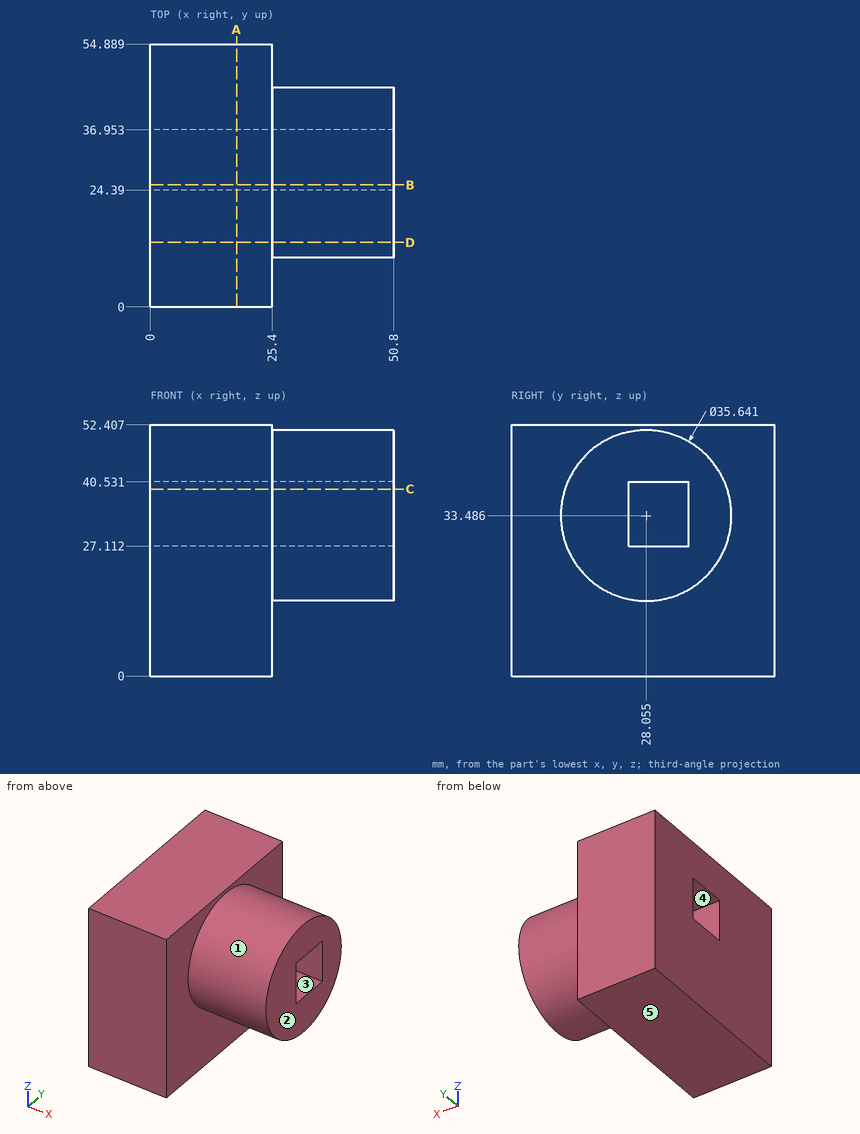
The drawing under review shows one solid part. Ordinate dimensions are in mm from its lowest x, y, z. A direction names the side the tool comes from. Round coordinates to 2 decimals unless told otherwise and drop trailing zeros. Order: outer loops, then holes, each group sorted by start corner. A loop starts at its lowest first (then second) coordinate and runs counter-clockwise, first axis right, second up. Notation, with made-up numbers: (-30, 6) -> (-2, 6) arc R21 ccw to (-2, 16) -> close; hole circle Ø4 at (-11, 1). An arc over 180 degrees is marked (long way). Return JSON: item names as keys, results as strings.
1. For the marked faces 4 and 5, list the 3-axis set-ups (+Z, -Z, +X, -X, +Y, -Y) from which the entire face can be reached by the end or side of a thin tool; tool diameter is ignored.
Answer block:
{"face 4": "+X, -X", "face 5": "-Z, +X, -X, +Y, -Y"}
2. The part is to be moulded in two halves that separate along Z. For the marked faces 1, 2 and 3, say which applies: +Z half, -Z half, draft (parallel to the pull), parting line (faces both ways), or undercut.
Answer block:
{"face 1": "parting line", "face 2": "draft", "face 3": "undercut"}
3. Take a section at B-B (y = 25.5). Write out the cut boundary in (x, z), then the cut area to 3 significant figures.
Answer block:
{"outline": "(0, 0) -> (25.4, 0) -> (25.4, 15.85) -> (50.8, 15.85) -> (50.8, 27.11) -> (0, 27.11) -> close; (0, 40.53) -> (50.8, 40.53) -> (50.8, 51.12) -> (25.4, 51.12) -> (25.4, 52.41) -> (0, 52.41) -> close", "area": "1,550 mm²"}
4. Take a section at D-D (y = 13.5). Write out the cut boundary in (x, z).
Answer block:
{"outline": "(0, 0) -> (25.4, 0) -> (25.4, 23.2) -> (50.8, 23.2) -> (50.8, 43.77) -> (25.4, 43.77) -> (25.4, 52.41) -> (0, 52.41) -> close"}
5. Take a section at C-C (z = 39). Write out the cut boundary in (x, y).
Answer block:
{"outline": "(0, 0) -> (25.4, 0) -> (25.4, 11.11) -> (50.8, 11.11) -> (50.8, 24.39) -> (0, 24.39) -> close; (0, 36.95) -> (50.8, 36.95) -> (50.8, 45) -> (25.4, 45) -> (25.4, 54.89) -> (0, 54.89) -> close"}
6. For L1, parallel to Z at x = 16, y = 27; L2, parallel to Y at x = 18, z = 28; L3, parallel to X at y = 49, z = 15.5, list the stretches that pass through material, from the lowest coordinate up. Write a range as [from, to].
Answer block:
{"L1": "z = [0, 27.11], [40.53, 52.41]", "L2": "y = [0, 24.39], [36.95, 54.89]", "L3": "x = [0, 25.4]"}
7. Insertion check: P1, Ø10, axis at x = 28.5, y = 32, coming from the +Z side; P2, Ø4, axis at x = 30, z = 31.5, coming from the -Y side (1 decimal); P3, Ø2, axis at y = 5.5, z = 11, coming from the +X side; P4, Ø1.5, axis at x = 45.5, y = 13.5, coming from the -Z side (1 decimal). Each pin has a flat end and moves straight along its axis. Give the tip position at first contact, or say it passes through.
Answer block:
{"P1": "stops at z = 52.41", "P2": "stops at y = 10.2", "P3": "stops at x = 25.4", "P4": "stops at z = 22.2"}
8. Take a section at A-A (x = 18). Write out the cut boundary in (y, z), then the cut area to 3 significant figures.
Answer block:
{"outline": "(0, 0) -> (54.89, 0) -> (54.89, 52.41) -> (0, 52.41) -> close; hole (24.39, 27.11) -> (36.95, 27.11) -> (36.95, 40.53) -> (24.39, 40.53) -> close", "area": "2,710 mm²"}
